The model under review builds one solid part; all positions refer to its coordinate system, in mm. Face numbers are marked on the shaded views. A direction names the side the tool comes from. Coordinates: 2 decimals unless noted, no trailing zeros. Loops run counter-clockwise (first coordinate to the right, second up) from the corner with the lowest first, then second, coordinate; pieces in that order, holes last. Notation, with made-up numbers: (50.25, 41.5) - (105.25, 41.5) arc R22 cw to (105.25, 66.5) - close; hole circle Ø4 at (79.25, 54.5). An arc over 180 degrees is marked (long way). One line per item, written item: value. Start each with the question number.
1. For the marked faces 4, 5, 6, 7 and 8, list the 3-axis set-ups (+Z, -Z, +X, -X, +Y, -Y) from which the entire face can be reached by the end or side of a thin tool; tool diameter is ignored.
2. To check wall thickness, follow line 1 (Z direction, x = -13.5, y = 4.5); line 2 (Z direction, x = -13, y = -1); line 3 (Y direction, x = 4, z = 2). State the ranges of each line that lie inside material, in increasing order.
3. We need section C-C, the plane x = 14.5. Give the boundary of the cut face in (y, z).
4. We need section A-A, the plane x = -13.5. Give the boundary of the cut face in (y, z).
5. Insertion check: P1, Ø8, axis at x = -20.5, z = 6, coming from the +Y side; P2, Ø0.6, axis at y = -9, z = 6.5, coming from the +X side; P3, Ø3, axis at x = 5.5, z = 18.5, coming from the -Y side. Each pin has a flat end and moves straight along its axis. Give the tip position at first contact, or say it passes through.
6. Mouldability with a two-part tool opening along X and no side actions: class the marked faces 1, 2 and 3 as +X half, -X half, draft (parallel to the pull), parting line (faces both ways), or undercut.
7. We need section B-B, the plane x = -21. Give the boundary of the cut face in (y, z) (3 decimals), then the cut area to 3 significant figures.
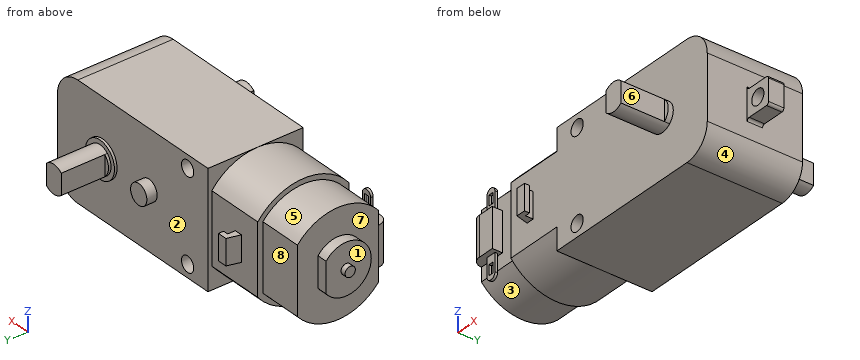
from build123d import *
from build123d import SkipClean  # not in build123d's __all__

# Parameters (mm, degrees)
F0_W           = 37
F0_H           = 18.6
F1_DEPTH       = 22.4
F3_DEPTH       = 11.3
F5_DEPTH       = 8.5
F7_DEPTH       = 2
F8_R           = 1
F9_DEPTH       = 1
F10_R          = 3.575
F11_DEPTH      = 0.5
F11_DEPTH_BACK = 19.1
F13_DEPTH      = 9
F13_DEPTH_BACK = 28.6
F14_R          = 5
F16_START      = -7.8
F15_W          = 5.25
F15_H          = 5.25
F15_R          = 1.5
F16_DEPTH      = 3
F17_R          = 0.5
F19_START      = -8.7
F19_DEPTH      = 5
F20_R          = 2
F21_DEPTH      = 2
F22_R          = 1.5
F23_DEPTH      = 28.101
F24_DEPTH      = 0.5
F25_R          = 2.725
F26_DEPTH      = 1
F26_DEPTH_BACK = 19.6
F27_W          = 5.2
F27_H          = 7.65
F28_DEPTH      = 2
F29_R          = 2
F31_START      = -1
F30_W          = 1
F30_H          = 2
F31_DEPTH      = 0.5


# Not quite as in the source:
# - after a boolean that leaves OpenCascade's solid faulty, fix() repairs it


with BuildPart() as f1:
    # F0 (on Top) → F1 (new body)
    with BuildSketch(Plane.XY):
        Rectangle(F0_W, F0_H)
    extrude(amount=F1_DEPTH)

    # F2 (on face) → F3 (join)
    with BuildSketch(Plane(origin=(-18.5, 0, 0), x_dir=(0, -1, 0), z_dir=(-1, 0, 0))):
        with BuildLine():
            ThreePointArc((-8.55, 4.35), (0.375, 0), (9.3, 4.35))
            Line((9.3, 4.35), (9.3, 18.05))
            ThreePointArc((9.3, 18.05), (0.375, 22.4), (-8.55, 18.05))
            Line((-8.55, 18.05), (-8.55, 4.35))
        make_face()
    extrude(amount=F3_DEPTH)

    # F4 (on face) → F5 (join)
    with BuildSketch(Plane(origin=(-29.8, 0, 0), x_dir=(0, -1, 0), z_dir=(-1, 0, 0))):
        with BuildLine():
            Line((-7.55, 17.6964123944), (-7.55, 4.7035876056))
            ThreePointArc((-7.55, 4.7035876056), (0.375, 1), (8.3, 4.7035876056))
            Line((8.3, 4.7035876056), (8.3, 17.6964123944))
            ThreePointArc((8.3, 17.6964123944), (0.375, 21.4), (-7.55, 17.6964123944))
        make_face()
    extrude(amount=F5_DEPTH)

    # F6 (on face) → F7 (join)
    with BuildSketch(Plane(origin=(-38.3, 0, 0), x_dir=(0, -1, 0), z_dir=(-1, 0, 0))):
        with BuildLine():
            Line((-3.525, 14.1664793948), (-3.525, 8.2335206052))
            ThreePointArc((-3.525, 8.2335206052), (5.275, 11.2), (-3.525, 14.1664793948))
        make_face()
    extrude(amount=F7_DEPTH)

    # F8 (on face) → F9 (join)
    with BuildSketch(Plane(origin=(-40.3, 0, 0), x_dir=(0, -1, 0), z_dir=(-1, 0, 0))):
        with Locations((0.375, 11.2)):
            Circle(F8_R)
    extrude(amount=F9_DEPTH)

    # F10 (on face) → F11 (join, two sides)
    with BuildSketch(Plane(origin=(0, 9.3, 0), x_dir=(-1, 0, 0), z_dir=(0, 1, 0))) as f11_sk:
        with Locations((-7.425, 11.2)):
            Circle(F10_R)
    extrude(amount=F11_DEPTH)
    extrude(f11_sk.sketch, amount=-F11_DEPTH_BACK)

    # F12 (on face) → F13 (join, two sides)
    with BuildSketch(Plane(origin=(0, 9.8, 0), x_dir=(-1, 0, 0), z_dir=(0, 1, 0))) as f13_sk:
        with BuildLine():
            Line((-5.6, 9.1763893655), (-5.6, 13.2236106345))
            ThreePointArc((-5.6, 13.2236106345), (-7.425, 13.925), (-9.25, 13.2236106345))
            Line((-9.25, 13.2236106345), (-9.25, 9.1763893655))
            ThreePointArc((-9.25, 9.1763893655), (-7.425, 8.475), (-5.6, 9.1763893655))
        make_face()
    extrude(amount=F13_DEPTH)
    extrude(f13_sk.sketch, amount=-F13_DEPTH_BACK)

    # F14
    f14_edges = [f1.edges().sort_by_distance(p)[0] for p in [
        (18.5, 0, 0),
        (18.5, 0, 22.4),
    ]]
    fillet(f14_edges, radius=F14_R)

    # F15 (on face) → F16 (join)
    with BuildSketch(Plane(origin=(0, 9.3, 0), x_dir=(-1, 0, 0), z_dir=(0, 1, 0)).offset(F16_START)):
        with Locations((-21.125, 11.2)):
            Rectangle(F15_W, F15_H)
        with Locations((-21.125, 11.2)):
            Circle(F15_R, mode=Mode.SUBTRACT)
    extrude(amount=-F16_DEPTH)

    # F17
    f17_edges = [f1.edges().sort_by_distance(p)[0] for p in [
        (23.75, 0, 13.825),
        (18.5, 0, 13.825),
        (23.75, 0, 8.575),
        (18.5, 0, 8.575),
    ]]
    fillet(f17_edges, radius=F17_R)

    # F18 (on face) → F19 (join)
    with BuildSketch(Plane.XY.offset(22.4).offset(F19_START)):
        Polygon((-25.1301270189, 11.05), (-25.8, 8.55), (-24.3, 8.55), (-24.3, 10.05), (-23.3, 10.05), (-23.3, 11.05), align=None)
        Polygon((-23.3, -10.8), (-24.3, -10.8), (-24.3, -9.3), (-25.8, -9.3), (-25.1301270189, -11.8), (-23.3, -11.8), align=None)
    extrude(amount=-F19_DEPTH)

    # F20 (on face) → F21 (join)
    with BuildSketch(Plane(origin=(0, 9.3, 0), x_dir=(-1, 0, 0), z_dir=(0, 1, 0))):
        with Locations((4, 11.2)):
            Circle(F20_R)
    extrude(amount=F21_DEPTH)

    # F22 (on face) → F23 (cut, through all)
    with BuildSketch(Plane(origin=(0, 9.3, 0), x_dir=(-1, 0, 0), z_dir=(0, 1, 0))):
        with Locations((13.5, 19.9)):
            Circle(F22_R)
        with Locations((13.5, 2.5)):
            Circle(F22_R)
    extrude(amount=-F23_DEPTH, mode=Mode.SUBTRACT)

    # F24 (cut): a face of the model
    f24_faces = [f1.faces().sort_by_distance(p)[0] for p in [
        (10.8988837303, -9.8, 11.2),
    ]]
    extrude(f24_faces, amount=-F24_DEPTH, mode=Mode.SUBTRACT)

    # F25 (on face) → F26 (join, two sides)
    with BuildSketch(Plane.XZ.offset(9.3)) as f26_sk:
        with Locations((7.425, 11.2)):
            Circle(F25_R)
    with SkipClean():  # cleaning this boolean's faces spoils the solid; the shape is the same uncleaned
        extrude(amount=F26_DEPTH)
        extrude(f26_sk.sketch, amount=-F26_DEPTH_BACK)

    # F27 (on face) → F28 (join)
    with BuildSketch(Plane.XZ.offset(8.3)):
        with Locations((-35.7, 11.2)):
            Rectangle(F27_W, F27_H)
    extrude(amount=F28_DEPTH)

    add(f1.part.fix(), mode=Mode.REPLACE)

    # F29
    f29_edges = [f1.edges().sort_by_distance(p)[0] for p in [
        (-38.3, -10.3, 11.2),
    ]]
    fillet(f29_edges, radius=F29_R)

    # F30 (on face) → F31 (join)
    with BuildSketch(Plane.XZ.offset(10.3).offset(F31_START)):
        with BuildLine():
            Line((-35.7, 18.525), (-35.7, 15.025))
            Line((-35.7, 15.025), (-33.7, 15.025))
            Line((-33.7, 15.025), (-33.7, 18.525))
            ThreePointArc((-33.7, 18.525), (-34.7, 19.525), (-35.7, 18.525))
        make_face()
        with Locations((-34.7, 17.525)):
            Rectangle(F30_W, F30_H, mode=Mode.SUBTRACT)
        with BuildLine():
            Line((-35.7, 7.375), (-35.7, 3.875))
            ThreePointArc((-35.7, 3.875), (-34.7, 2.875), (-33.7, 3.875))
            Line((-33.7, 3.875), (-33.7, 7.375))
            Line((-33.7, 7.375), (-35.7, 7.375))
        make_face()
        with Locations((-34.7, 4.875)):
            Rectangle(F30_W, F30_H, mode=Mode.SUBTRACT)
    extrude(amount=-F31_DEPTH)


solid = f1.part
Findings below:
1. face 4: -Z, +X, +Y, -Y
1. face 5: +Z, -X
1. face 6: +Z, -Z, +X, -Y
1. face 7: -X
1. face 8: +Z, -Z, -X, +Y
2. line 1: 0 to 1, 4 to 18.4, 21.4 to 22.4
2. line 2: 0 to 1.09, 3.91 to 18.49, 21.31 to 22.4
2. line 3: -9.3 to 9.3
3. outline: (-9.3, 0.1) - (9.3, 0.1) - (9.3, 22.3) - (-9.3, 22.3) - close
4. outline: (-9.3, 0) - (9.3, 0) - (9.3, 1) - (-9.3, 1) - close; (-9.3, 4) - (9.3, 4) - (9.3, 18.4) - (-9.3, 18.4) - close; (-9.3, 21.4) - (9.3, 21.4) - (9.3, 22.4) - (-9.3, 22.4) - close
5. P1: y = 11.05
5. P2: x = 18.5
5. P3: y = -9.3
6. face 1: -X half
6. face 2: undercut
6. face 3: draft
7. outline: (-9.3, 4.35) arc R11.331 ccw to (8.55, 4.35) - (8.55, 18.05) arc R11.331 ccw to (-9.3, 18.05) - close
7. area: 353 mm2
